Verification items for the finished model (mm, model axes). A direction names the side the tool comes from. Round coordinates to 2 decimals unless told otherwise and drop trailing zeros. Write each loop counter-clockwise with the first axis right and the second up, starting at its lowest first coordinate (ties: lowest second). Pieces come first, ordered by that corner, then holes.
from build123d import *

# Parameters (mm, degrees)
BOSS_EXTRUDE1_DEPTH      = 3.5814
SKETCH7_W                = 39.878
SKETCH7_H                = 24
BOSS_EXTRUDE2_DEPTH      = 3.035
BOSS_EXTRUDE2_DEPTH_BACK = 3.035
SKETCH5_R                = 5
SKETCH5_R_2              = 1.45
SKETCH5_RX               = 8
SKETCH5_RY               = 4
CUT_EXTRUDE3_DEPTH       = 1
CUT_EXTRUDE3_DEPTH_BACK  = 7.6164
SKETCH8_W                = 18.796
SKETCH8_H                = 3.035
CUT_EXTRUDE4_DEPTH       = 10


with BuildPart() as part:
    # Sketch1 → Boss-Extrude1 (new body)
    with BuildSketch(Plane(origin=(0, 0, 0), x_dir=(1, 0, 0), z_dir=(0, 1, 0))):
        Polygon((-12.79, -26.1874988), (27.088, -26.1874988), (27.088, -2.1874988), (1.7907, -2.1874988), (1.7907, 2.1874988), (9.398, 2.1874988), (1.7907, 7.2674988), (-1.7907, 7.2674988), (-9.398, 2.1874988), (-1.7907, 2.1874988), (-1.7907, -2.1874988), (-12.79, -2.1874988), align=None)
    extrude(amount=BOSS_EXTRUDE1_DEPTH)

    # Sketch7 → Boss-Extrude2 (add, two sides)
    with BuildSketch(Plane(origin=(0, 0, 0), x_dir=(1, 0, 0), z_dir=(0, 1, 0))) as boss_extrude2_sk:
        with Locations((7.149, -14.1874988)):
            Rectangle(SKETCH7_W, SKETCH7_H)
    extrude(amount=BOSS_EXTRUDE2_DEPTH)
    extrude(boss_extrude2_sk.sketch, amount=-BOSS_EXTRUDE2_DEPTH_BACK)

    # Sketch5 → Cut-Extrude3 (cut, two sides)
    with BuildSketch(Plane(origin=(0, 3.5814, 0), x_dir=(1, 0, 0), z_dir=(0, 1, 0))) as cut_extrude3_sk:
        with Locations((-0.79, -14.1874988)):
            Circle(SKETCH5_R)
        with Locations((19.738, -22.6964988)):
            Circle(SKETCH5_R_2)
        with Locations((19.738, -5.6784988)):
            Circle(SKETCH5_R_2)
        with Locations(Location((7.21, -14.1874988), (0, 0, 180))):
            Ellipse(SKETCH5_RX, SKETCH5_RY)
    extrude(amount=CUT_EXTRUDE3_DEPTH, mode=Mode.SUBTRACT)
    extrude(cut_extrude3_sk.sketch, amount=-CUT_EXTRUDE3_DEPTH_BACK, mode=Mode.SUBTRACT)

    # Sketch8 → Cut-Extrude4 (cut)
    with BuildSketch(Plane(origin=(0, 0, 2.1874988), x_dir=(-1, 0, 0), z_dir=(0, 0, -1))):
        with Locations((0, -1.5175)):
            Rectangle(SKETCH8_W, SKETCH8_H)
    extrude(amount=-CUT_EXTRUDE4_DEPTH, mode=Mode.SUBTRACT)


solid = part.part
Q1. Material ranges on line 1 along Z through (x, y) = (19.5, 3.25); line 2 along Z through (x, y) = (-4.5, 1.25); line 3 along Z through (x, y) = (-0.79, 0.5), recorded low to high.
Recorded:
line 1: z = 2.19 to 4.25, 7.11 to 21.27, 24.13 to 26.19
line 2: z = -5.46 to -2.19, 2.19 to 10.84, 17.54 to 26.19
line 3: z = -7.27 to 9.19, 19.19 to 26.19
Q2. Release check for a two-part mould opening along Z. For faces 6 (the flat face through (6, 2, -2.187)), 7 (the flat face through (0, 0, 4)), 8 (the flat face through (-7, -1, 12.187)), 9 (the flat face through (1.791, 2, 0)) record: released by +Z, released by -Z, zero draft, split by the parting line, or undercut.
Recorded:
face 6: undercut
face 7: zero draft
face 8: released by -Z
face 9: undercut
Q3. Tool access check on faces 1 (the flat face through (-6, 2, -2.187)), 2 (the flat face through (17, 0, 2.187)), 3 (the flat face through (9.398, -2, 6)), 4 (the flat face through (0, 2, -7.267)), 5 (the flat face through (-12.79, 0, 14)). Record the directions out of +Z, -Z, +X, -X, +Y, -Y that give a thin tool (end or side, any length) a straight path to the whole face; none if there is none.
Recorded:
face 1: -X, +Y, -Y
face 2: +X, +Y, -Y
face 3: -Z, -Y
face 4: -Z, +X, -X, +Y, -Y
face 5: +Z, -Z, -X, +Y, -Y
Q4. Depth check by flat-ended pin: P1, Ø3, axis at y = 2, z = -0.5, coming from the -X side; P2, Ø1.8, axis at y = 2.5, z = 0, coming from the +X side; P3, Ø2, axis at x = 5, z = 10, coming from the -Y side; P4, Ø1, axis at x = -7.5, z = 1, coming from the -Y side. Enter the tip coordinate at first touch or a pass-through.
Recorded:
P1: stops at x = -1.79
P2: stops at x = 1.79
P3: stops at y = 0
P4: passes through
Q5. Sectioned sample at B-B (z = 5). Enter the section's corners in (x, y) (3 decimals), plus the area to 3 significant figures.
Recorded:
outline: (-12.79, -3.035) - (-9.398, -3.035) - (-9.398, 0) - (9.398, 0) - (9.398, -3.035) - (18.457, -3.035) - (18.457, 3.581) - (-12.79, 3.581) - close; (21.019, -3.035) - (27.088, -3.035) - (27.088, 3.581) - (21.019, 3.581) - close
area: 190 mm2
Q6. Sectioned sample at D-D (z = -3). Enter the section's corners in (x, y), plus the area to 3 significant figures.
Recorded:
outline: (-8.18, 0) - (8.18, 0) - (8.18, 3.58) - (-8.18, 3.58) - close
area: 58.6 mm2
Q7. Sectioned sample at A-A (x = -0.79). Enter the section's corners in (y, z) (1 decimal), plus the area to 3 significant figures.
Recorded:
outline: (-3, 19.2) - (3.6, 19.2) - (3.6, 26.2) - (-3, 26.2) - close; (0, -7.3) - (3.6, -7.3) - (3.6, 9.2) - (0, 9.2) - close
area: 105 mm2
Q8. Sectioned sample at C-C (x = 7). Give the number of separate pieces and of enclosed holes in the cut face, plus the area to 3 significant figures.
Recorded:
separate pieces: 3
enclosed holes: 0
area: 87.3 mm2
